from build123d import *

# Parameters (mm, degrees)
SKETCH2_R               = 3
BOSS_EXTRUDE1_DEPTH     = 180
CUT_EXTRUDE1_DEPTH      = 351.0628515
CUT_EXTRUDE1_DEPTH_BACK = 351.0628515
SKETCH3_W               = 50
SKETCH3_H               = 290
CUT_EXTRUDE2_DEPTH      = 351.0628515
CUT_EXTRUDE2_DEPTH_BACK = 351.0628515
SKETCH5_W               = 159.12266695
SKETCH5_H               = 409.499518343
SKETCH8_R               = 4
BOSS_EXTRUDE3_DEPTH     = 5
SKETCH9_R               = 1.5
CUT_EXTRUDE4_DEPTH      = 5


with BuildPart() as part:
    # Sketch2 → Boss-Extrude1 (new body)
    with BuildSketch(Plane(origin=(0, 0, 0), x_dir=(0, 0, -1), z_dir=(1, 0, 0))):
        with BuildLine():
            Line((159.16515139, 5), (265.83484861, 5))
            ThreePointArc((265.83484861, 5), (275, 12), (284.16515139, 5))
            Line((284.16515139, 5), (300, 5))
            Line((300, 5), (300, 0))
            Line((300, 0), (284.16515139, 0))
            ThreePointArc((284.16515139, 0), (275, -7), (265.83484861, 0))
            Line((265.83484861, 0), (159.16515139, 0))
            ThreePointArc((159.16515139, 0), (150, -7), (140.83484861, 0))
            Line((140.83484861, 0), (34.16515139, 0))
            ThreePointArc((34.16515139, 0), (25, -7), (15.83484861, 0))
            Line((15.83484861, 0), (0, 0))
            Line((0, 0), (0, 5))
            Line((0, 5), (15.83484861, 5))
            ThreePointArc((15.83484861, 5), (25, 12), (34.16515139, 5))
            Line((34.16515139, 5), (140.83484861, 5))
            ThreePointArc((140.83484861, 5), (150, 12), (159.16515139, 5))
        make_face()
        with Locations(Location((150, 2.5, 0), (0, 0, 180))):
            Circle(SKETCH2_R, mode=Mode.SUBTRACT)
        with Locations(Location((275, 2.5, 0), (0, 0, 180))):
            Circle(SKETCH2_R, mode=Mode.SUBTRACT)
        with Locations(Location((25, 2.5, 0), (0, 0, 180))):
            Circle(SKETCH2_R, mode=Mode.SUBTRACT)
    extrude(amount=BOSS_EXTRUDE1_DEPTH)

    # Sketch3 → Cut-Extrude1 (cut, two sides: drawn at the far end of the back side and taken through both)
    with BuildSketch(Plane(origin=(0, 5, 0), x_dir=(1, 0, 0), z_dir=(0, 1, 0)).offset(-CUT_EXTRUDE1_DEPTH_BACK)):
        with Locations((150, 150)):
            Rectangle(SKETCH3_W, SKETCH3_H)
        with Locations((90, 150)):
            Rectangle(SKETCH3_W, SKETCH3_H)
        with Locations((30, 150)):
            Rectangle(SKETCH3_W, SKETCH3_H)
    extrude(amount=CUT_EXTRUDE1_DEPTH + CUT_EXTRUDE1_DEPTH_BACK, mode=Mode.SUBTRACT)

    # Sketch5 → Cut-Extrude2 (cut, two sides: drawn at the far end of the back side and taken through both)
    with BuildSketch(Plane(origin=(0, 5, 0), x_dir=(1, 0, 0), z_dir=(0, 1, 0)).offset(-CUT_EXTRUDE2_DEPTH_BACK)):
        with Locations((139.561333475, 139.935321467)):
            Rectangle(SKETCH5_W, SKETCH5_H)
    extrude(amount=CUT_EXTRUDE2_DEPTH + CUT_EXTRUDE2_DEPTH_BACK, mode=Mode.SUBTRACT)

    # Sketch8 → Boss-Extrude3 (add)
    with BuildSketch(Plane(origin=(0, 0, 0), x_dir=(-1, 0, 0), z_dir=(0, -1, 0))):
        with Locations((-57.5, 48)):
            Circle(SKETCH8_R)
        with BuildLine():
            Line((-25, -1.5), (-35, -1.5))
            ThreePointArc((-35, -1.5), (-39, 2.5), (-35, 6.5))
            Line((-35, 6.5), (-25, 6.5))
            ThreePointArc((-25, 6.5), (-21, 2.5), (-25, -1.5))
        make_face()
        with BuildLine():
            Line((-2.475564239, 44), (-2.475564239, 52))
            ThreePointArc((-2.475564239, 52), (-6.475564239, 48), (-2.475564239, 44))
        make_face()
    extrude(amount=-BOSS_EXTRUDE3_DEPTH)

    # Sketch9 → Cut-Extrude4 (cut)
    with BuildSketch(Plane(origin=(0, 0, 0), x_dir=(-1, 0, 0), z_dir=(0, -1, 0))):
        with Locations(Location((-25, 3, 0), (0, 0, 90))):
            Circle(SKETCH9_R)
        with Locations(Location((-35, 3, 0), (0, 0, 90))):
            Circle(SKETCH9_R)
        with Locations(Location((-57.5, 48, 0), (0, 0, 90))):
            Circle(SKETCH9_R)
        with Locations(Location((-2.5, 48, 0), (0, 0, 90))):
            Circle(SKETCH9_R)
    extrude(amount=-CUT_EXTRUDE4_DEPTH, mode=Mode.SUBTRACT)


solid = part.part
CAD build for the part. Positions are in the model's coordinates, mm. A direction names the side the tool comes from. Give positions to 0.01 mm unless a question says otherwise; leave off trailing zeros. Write each loop counter-clockwise with the first axis right and the second up, starting at its lowest first coordinate (ties: lowest second). Pieces come first, ordered by that corner, then holes. Notation, with made-up numbers: (52, 21.5) -> (109, 21.5) arc R8 cw to (109, 27.5) -> close; hole circle Ø6 at (24.25, -7.5). An arc over 180 degrees is marked (long way). Return JSON: item names as keys, results as strings.
Item 1: Drop flat-ended pins along their axis: pin 1 (5 mm diameter, centred on x = 2.5, z = -74, fed in from -Y); pin 2 (8 mm diameter, centred on x = 53.5, y = 3.5, fed in from +Z); pin 3 (8 mm diameter, centred on y = 4.5, z = -231, fed in from +X); pin 4 (12 mm diameter, centred on x = 16.5, z = -42.5, fed in from +Y). Give the stop position or say it passes through.
Answer below:
{"pin 1": "stops at y = 0", "pin 2": "stops at z = 0", "pin 3": "stops at x = 60", "pin 4": "passes through"}
Item 2: Band-saw the part on C-C (y = 2.5). Give the number of separate pieces and of enclosed holes in the cut face, then the cut area to 3 significant figures.
Answer below:
{"separate pieces": "6", "enclosed holes": "4", "area": "3,350 mm2"}
Item 3: Tool access for faces 4 (the flat face through (2, 0, -88)), 5 (the flat face through (5, 2, -171)), 6 (the flat face through (30, 0, -296)): list every direction of +Z, -Z, +X, -X, +Y, -Y with a clear straight run to the whole face (end or side of a thin tool).
Answer below:
{"face 4": "+X, -X, -Y", "face 5": "+Y, -Y", "face 6": "-Z, +X, -X, -Y"}
Item 4: Drill centre lines: probe 1 along X at (y, z) = (3.3, -3); probe 2 along Z at (x, y) = (20.5, 4); probe 3 along X at (y, z) = (-0.75, -281.5). Where is each one in solid material? Low to high.
Answer below:
{"probe 1": "x = 0 to 23.5, 26.5 to 33.5, 36.5 to 60", "probe 2": "z = -300 to -295, -5 to 0", "probe 3": "x = 0 to 5, 55 to 60"}
Item 5: Two-plate mould, pull along X, no slides. Class faces 1 (the cylindrical face through (53.5, 2.5, -47.9)), 2 (the flat face through (2, 5, -212)), 3 (the cylindrical face through (61.5, 2.5, -48.1)): +X half, -X half, draft (parallel to the pull), parting line (faces both ways), or undercut.
Answer below:
{"face 1": "undercut", "face 2": "draft", "face 3": "+X half"}
Item 6: Band-saw the part on B-B (x = 43.5). List the corners of the cut face in (y, z), then the cut area to 3 significant figures.
Answer below:
{"outline": "(0, -300) -> (5, -300) -> (5, -295) -> (0, -295) -> close; (0, -5) -> (5, -5) -> (5, 0) -> (0, 0) -> close", "area": "50.0 mm2"}
Item 7: Band-saw the part on A-A (z = -199). List the corners of the cut face in (x, y), then the cut area to 3 significant figures.
Answer below:
{"outline": "(0, 0) -> (5, 0) -> (5, 5) -> (0, 5) -> close; (55, 0) -> (60, 0) -> (60, 5) -> (55, 5) -> close", "area": "50.0 mm2"}
